Design review of the part built by this model. Coordinates are the model's own, in mm. A direction names the side the tool comes from. Coordinates: 2 decimals unless noted, no trailing zeros. Write each loop counter-clockwise with the first axis right and the second up, starting at its lowest first coordinate (ties: lowest second). Pieces come first, ordered by that corner, then holes. Notation, with made-up numbers: (5, 49.5) -> (39, 49.5) arc R17 cw to (39, 70.5) -> close; hole circle Ø11 at (-14, -1.5). An arc over 180 degrees is marked (long way). Return JSON: item names as keys, results as strings. Group by question number.
from build123d import *

# Parameters (mm, degrees)
F0_W     = 10
F0_H     = 75
F1_DEPTH = 100
F3_D     = 5
F3_DEPTH = 15
F3_TIP   = 1.5021515476
F4_R     = 5
F5_DEPTH = 10
F7_DEPTH = 10


with BuildPart() as f1:
    # F0 (on Top) → F1 (new body)
    with BuildSketch(Plane.XY):
        Rectangle(F0_W, F0_H)
    extrude(amount=F1_DEPTH)

    # F3
    with Locations(Plane(origin=(0, 0, 0), x_dir=(1, 0, 0), z_dir=(0, 0, -1))):
        with Locations((0, 25), (0, -25)):
            Hole(F3_D / 2, depth=F3_DEPTH)
            with Locations((0, 0, -(F3_DEPTH + F3_TIP / 2))):  # 118° drill point
                Cone(0, F3_D / 2, F3_TIP, mode=Mode.SUBTRACT)

    # F4 (on face) → F5 (cut, through all)
    with BuildSketch(Plane(origin=(-5, 0, 0), x_dir=(0, -1, 0), z_dir=(-1, 0, 0))):
        with Locations((0, 50)):
            Circle(F4_R)
    extrude(amount=-F5_DEPTH, mode=Mode.SUBTRACT)

    # F6 (on face) → F7 (cut, through all)
    with BuildSketch(Plane(origin=(-5, 0, 0), x_dir=(0, -1, 0), z_dir=(-1, 0, 0))):
        with BuildLine():
            ThreePointArc((-21.6506350946, 37.5), (-25, 50), (-21.6506350946, 62.5))
            ThreePointArc((-21.6506350946, 62.5), (-23.4807621135, 69.3301270189), (-30.3108891325, 67.5))
            ThreePointArc((-30.3108891325, 67.5), (-35, 50), (-30.3108891325, 32.5))
            ThreePointArc((-30.3108891325, 32.5), (-23.4807621135, 30.6698729811), (-21.6506350946, 37.5))
        make_face()
    extrude(amount=-F7_DEPTH, mode=Mode.SUBTRACT)


solid = f1.part
Q1. Wall thickness on L1, parallel to Y at x = 0.25, z = 14; L2, parallel to X at y = -25, z = 8; L3, parallel to Y at x = -2.75, z = 52: over which ranges is each line inside the solid? List them lowest first.
Q2. For P1, Ø1.5, axis at x = 0, y = 7, coming from the -Z side; P2, Ø4, axis at x = 0, y = -25, coming from the -Z side, all flat-tipped, find the tip position at first contact; note any pin that passes through.
Q3. The part is to be moulded in two halves that separate along Y. For faces 1 (the cylindrical face through (-0.07, 0.651, 54.957)), 2 (the flat face through (0, -37.5, 49)), 3 (the cylindrical face through (-0.07, 23.386, 69.274)), 4 (the flat face through (0, 1, 0)), say which applies: +Y half, -Y half, draft (parallel to the pull), parting line (faces both ways), or undercut.
Q4. For faces 5 (the cylindrical face through (0, 25, 50)), 6 (the flat face through (-5, -9, 49)), 7 (the cylindrical face through (0.33, 22.52, 7.6)), list the 3-axis set-ups (+Z, -Z, +X, -X, +Y, -Y) from which the entire face can be reached by the end or side of a thin tool; tool diameter is ignored.
Q5. We need section A-A on z = 50. Write out the cut boundary in (x, y).
Q6. We need section D-D on z = 65. Write out the cut boundary in (x, y).
Q7. We need section C-C on y = 0. Write out the cut boundary in (x, z), plus the area to 3 significant figures.
Q8. We need section B-B on x = -3.75. Write out the cut boundary in (y, z).
Findings below:
{
 "1": {"L1": "y = -37.5 to -27.49, -22.51 to 22.51, 27.49 to 37.5", "L2": "x = -5 to -2.5, 2.5 to 5", "L3": "y = -37.5 to -4.58, 4.58 to 24.92, 34.94 to 37.5"},
 "2": {"P1": "stops at z = 0", "P2": "stops at z = 15.3"},
 "3": {"face 1": "undercut", "face 2": "-Y half", "face 3": "undercut", "face 4": "draft"},
 "4": {"face 5": "+X, -X", "face 6": "+Z, -Z, -X, +Y, -Y", "face 7": "-Z"},
 "5": {"outline": "(-5, -37.5) -> (5, -37.5) -> (5, -5) -> (-5, -5) -> close; (-5, 5) -> (5, 5) -> (5, 25) -> (-5, 25) -> close; (-5, 35) -> (5, 35) -> (5, 37.5) -> (-5, 37.5) -> close"},
 "6": {"outline": "(-5, -37.5) -> (5, -37.5) -> (5, 20.98) -> (-5, 20.98) -> close; (-5, 31.62) -> (5, 31.62) -> (5, 37.5) -> (-5, 37.5) -> close"},
 "7": {"outline": "(-5, 0) -> (5, 0) -> (5, 45) -> (-5, 45) -> close; (-5, 55) -> (5, 55) -> (5, 100) -> (-5, 100) -> close", "area": "900 mm^2"},
 "8": {"outline": "(-37.5, 0) -> (37.5, 0) -> (37.5, 100) -> (-37.5, 100) -> close; hole circle Ø10 at (0, 50); hole (21.65, 37.5) arc R5 ccw to (30.31, 32.5) arc R35 ccw to (30.31, 67.5) arc R5 ccw to (21.65, 62.5) arc R25 cw to start"}
}
